```python
from build123d import *

# Parameters (mm, degrees)
SKETCH014_W  = 3.21
SKETCH014_H  = 3.21
PAD012_DEPTH = 0.18
SKETCH013_W  = 2.63
SKETCH013_H  = 2.6
PAD011_DEPTH = 3
SKETCH011_W  = 7.6
SKETCH011_H  = 6.6
PAD010_DEPTH = 3.6
SKETCH012_W  = 6.16
SKETCH012_H  = 5.02
POCKET_DEPTH = 3.05


with BuildPart() as body012:
    # Sketch014 → Pad012 (new body)
    with BuildSketch(Plane.XY):
        with Locations((-0.565, -15.485)):
            Rectangle(SKETCH014_W, SKETCH014_H)
    extrude(amount=PAD012_DEPTH)


with BuildPart() as body012_1:
    # Body012 placement: moved
    add(body012.part.moved(Location((0, 0, 3.04))))


with BuildPart() as obj1:
    # Sketch013 → Pad011 (new body)
    with BuildSketch(Plane.XY):
        with Locations((-0.565, -15.48)):
            Rectangle(SKETCH013_W, SKETCH013_H)
    extrude(amount=PAD011_DEPTH)


with BuildPart() as obj1_1:
    # Body011 placement: moved
    add(obj1.part.moved(Location((0, 0, 1.92))))


with BuildPart() as cut001_outer_shell:
    # Sketch011 → Pad010 (new body)
    with BuildSketch(Plane.XY):
        with Locations((0, -15.37)):
            Rectangle(SKETCH011_W, SKETCH011_H)
    extrude(amount=PAD010_DEPTH)

    # Sketch012 → Pocket (cut)
    with BuildSketch(Plane.XY):
        with Locations((-0.02, -15.33)):
            Rectangle(SKETCH012_W, SKETCH012_H)
    extrude(amount=POCKET_DEPTH, mode=Mode.SUBTRACT)

    # Cut: cut obj1
    add(obj1_1.part, mode=Mode.SUBTRACT)

    # Cut001: cut Body012
    add(body012_1.part, mode=Mode.SUBTRACT)


solid = cut001_outer_shell.part
```
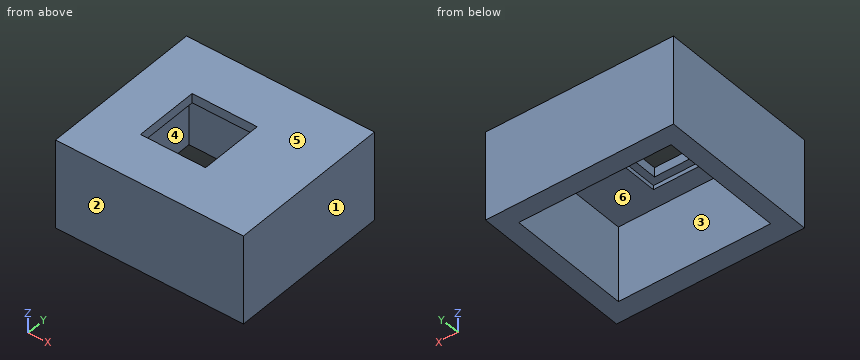
Build history of the part. All positions in model axes, mm. Face numbers are marked on the shaded views. A direction names the side the tool comes from. Give positions to 0.01 mm unless a question says otherwise; leave off trailing zeros. Loops run counter-clockwise (first coordinate to the right, second up) from the corner with the lowest first, then second, coordinate; pieces in that order, holes last. Notation, with made-up numbers: (-5.75, 12.25) -> (53.25, 12.25) arc R35 ccw to (53.25, 48.25) -> close; hole circle Ø1 at (88.25, -13.75). An arc over 180 degrees is marked (long way). One line per question, with ' | ' between items. Start each with the question number.
1) Cut at B-B (x = 0.25). Give the cut face in (y, z).
2) Two-plate mould, pull along X, no slides. Class the marked faces 1, 2, 3 and 4: released by +X, released by -X, zero draft, split by the parting line, or undercut.
3) Cut at A-A (y = -16). Give the cut face in (x, z).
4) 3-axis set-ups, long thin cutter, end or side, ignore diameter. For the marked faces 5 and 6: which of +Z, -Z, +X, -X, +Y, -Y reach the whole face in a straight line?
5) Pin check, flat tip, straight feed: pin 1 (3.5 mm diameter, centred on x = -1, y = -16, fed in from -Z). Stop position of the tip, or through.
6) Probe L1, parallel to Y at x = -1, z = 1.3; L2, parallel to X at y = -16, z = 2.3; L3, parallel to X at y = -17, z = 3.15. List the from-to ranges inside material, lowest first.
7) Cut at D-D (y = -17). Give the cut face in (x, z).
8) Cut at C-C (z = 0.9). Give the cut face in (x, y).
Return value:
1) outline: (-18.67, 0) -> (-17.84, 0) -> (-17.84, 3.05) -> (-17.09, 3.05) -> (-17.09, 3.22) -> (-16.78, 3.22) -> (-16.78, 3.6) -> (-18.67, 3.6) -> close; (-14.18, 3.22) -> (-13.88, 3.22) -> (-13.88, 3.05) -> (-12.82, 3.05) -> (-12.82, 0) -> (-12.07, 0) -> (-12.07, 3.6) -> (-14.18, 3.6) -> close
2) face 1: released by +X | face 2: zero draft | face 3: undercut | face 4: undercut
3) outline: (-3.8, 0) -> (-3.1, 0) -> (-3.1, 3.05) -> (-2.17, 3.05) -> (-2.17, 3.22) -> (-1.88, 3.22) -> (-1.88, 3.6) -> (-3.8, 3.6) -> close; (0.75, 3.22) -> (1.04, 3.22) -> (1.04, 3.05) -> (3.06, 3.05) -> (3.06, 0) -> (3.8, 0) -> (3.8, 3.6) -> (0.75, 3.6) -> close
4) face 5: +Z, +X, -X, +Y, -Y | face 6: -Z
5) pin 1: z = 3.05
6) L1: -18.67 to -17.84, -12.82 to -12.07 | L2: -3.8 to -3.1, 3.06 to 3.8 | L3: -3.8 to -2.17, 1.04 to 3.8
7) outline: (-3.8, 0) -> (-3.1, 0) -> (-3.1, 3.05) -> (-2.17, 3.05) -> (-2.17, 3.22) -> (1.04, 3.22) -> (1.04, 3.05) -> (3.06, 3.05) -> (3.06, 0) -> (3.8, 0) -> (3.8, 3.6) -> (-3.8, 3.6) -> close
8) outline: (-3.8, -18.67) -> (3.8, -18.67) -> (3.8, -12.07) -> (-3.8, -12.07) -> close; hole (-3.1, -17.84) -> (3.06, -17.84) -> (3.06, -12.82) -> (-3.1, -12.82) -> close
